Source: three-view drawing plus pictorial views. Frame: mm from the lowest corner of the part. A direction names the side the tool comes from. Give positions to 0.01 mm unless a question says otherwise; leave off trailing zeros. Loops run counter-clockwise (first coordinate to the right, second up) from the corner with the lowest first, then second, coordinate; pieces in that order, holes last. Notation, with made-up numbers: (46.5, 59.25) - (61.5, 59.25) arc R33 cw to (61.5, 92.25) - close; hole circle Ø1 at (83, 2). An arc over 180 degrees is marked (long way). Answer in a Markdown table with one row per item.
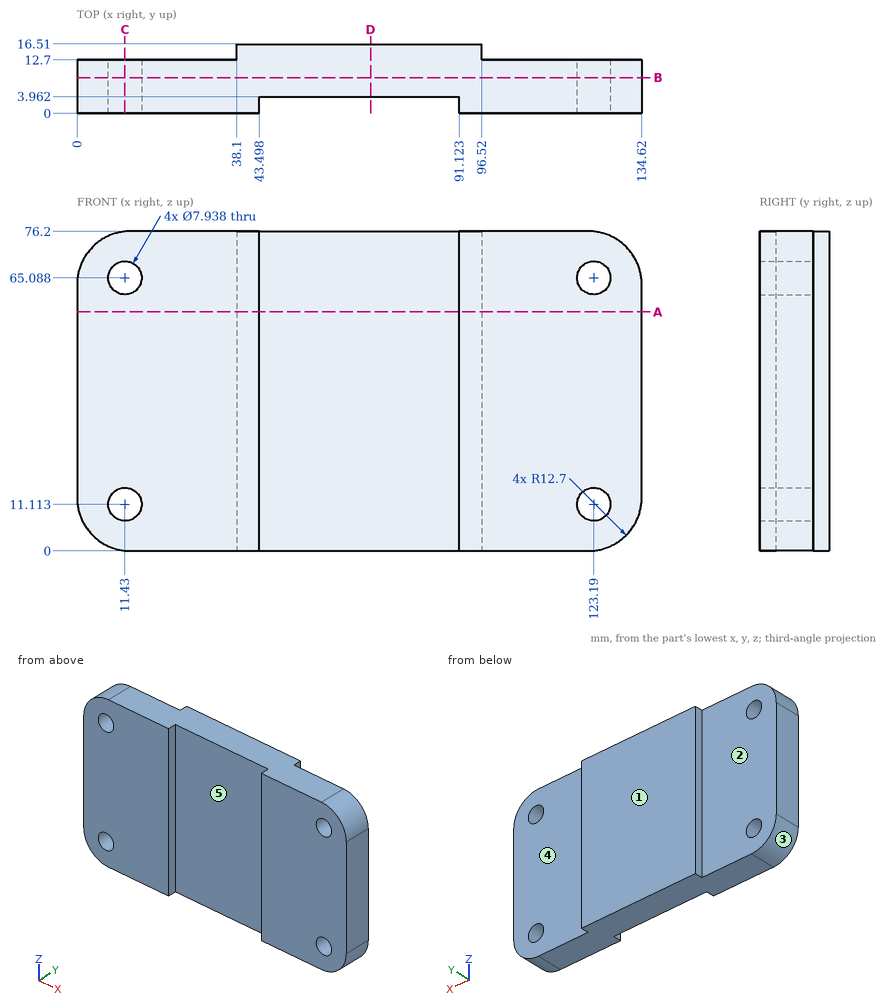
Q1. Cut plane A-A (z = 57). Output: boundary loops of the cut face in (x, y), and give its area (3 significant figures).
Check values:
| item | result |
|---|---|
| outline | (0, 0) - (43.5, 0) - (43.5, 3.96) - (91.12, 3.96) - (91.12, 0) - (134.62, 0) - (134.62, 12.7) - (96.52, 12.7) - (96.52, 16.51) - (38.1, 16.51) - (38.1, 12.7) - (0, 12.7) - close |
| area | 1,740 mm² |
Q2. Cut plane D-D (x = 70). Output: boundary loops of the cut face in (y, z), and give its area (3 significant figures).
Check values:
| item | result |
|---|---|
| outline | (3.96, 0) - (16.51, 0) - (16.51, 76.2) - (3.96, 76.2) - close |
| area | 956 mm² |
Q3. Draft query along X for the marked faces 3, 4 and 5. Return one class per face: pulls with the +X half, pulls with the -X half, needs draft (parallel to the pull), parting line crosses it, or undercut.
Check values:
| item | result |
|---|---|
| face 3 | pulls with the -X half |
| face 4 | needs draft |
| face 5 | undercut |
Q4. Material intervals for line 1 along X through (y, z) = (1, 17); line 2 along Z through (x, y) = (9.5, 11.5) (1 decimal); line 3 along Z through (x, y) = (123.19, 3), sorted ascending.
Check values:
| item | result |
|---|---|
| line 1 | 0 to 43.5, 91.12 to 134.62 |
| line 2 | 0.4 to 7.6, 14.6 to 61.6, 68.6 to 75.8 |
| line 3 | 0.06 to 7.14, 15.08 to 61.12, 69.06 to 76.14 |
Q5. First-contact query: pin 1 (19 mm diameter, centred on x = 112.5, z = 30.5, fed in from +Y); pin 2 (1.5 mm diameter, centred on y = 9.5, z = 9, fed in from -X); pin 3 (6.5 mm diameter, centred on x = 123.19, z = 11.11, fed in from -Y); pin 4 (1.1 mm diameter, centred on y = 15.5, z = 31.5, fed in from -X). Flat tips, straight axial feed; report the tip coordinate or a pass-through.
Check values:
| item | result |
|---|---|
| pin 1 | y = 12.7 |
| pin 2 | x = 0.35 |
| pin 3 | through |
| pin 4 | x = 38.1 |
Q6. Cut plane B-B (y = 8.5). Output: boundary loops of the cut face in (x, z).
Check values:
| item | result |
|---|---|
| outline | (0, 12.7) arc R12.7 ccw to (12.7, 0) - (121.92, 0) arc R12.7 ccw to (134.62, 12.7) - (134.62, 63.5) arc R12.7 ccw to (121.92, 76.2) - (12.7, 76.2) arc R12.7 ccw to (0, 63.5) - close; hole circle Ø7.94 at (11.43, 11.11); hole circle Ø7.94 at (11.43, 65.09); hole circle Ø7.94 at (123.19, 11.11); hole circle Ø7.94 at (123.19, 65.09) |
Q7. Reachability of the marked faces 1 and 2 from +Z, -Z, +X, -X, +Y, -Y: full face, straight path, thin tool, end or side. Return the list, or none.
Check values:
| item | result |
|---|---|
| face 1 | +Z, -Z, +X, -X, +Y |
| face 2 | +Z, -Z, -X, +Y |
Q8. Cut plane C-C (x = 11.43). Output: boundary loops of the cut face in (y, z).
Check values:
| item | result |
|---|---|
| outline | (0, 0.06) - (12.7, 0.06) - (12.7, 7.14) - (0, 7.14) - close; (0, 15.08) - (12.7, 15.08) - (12.7, 61.12) - (0, 61.12) - close; (0, 69.06) - (12.7, 69.06) - (12.7, 76.14) - (0, 76.14) - close |
